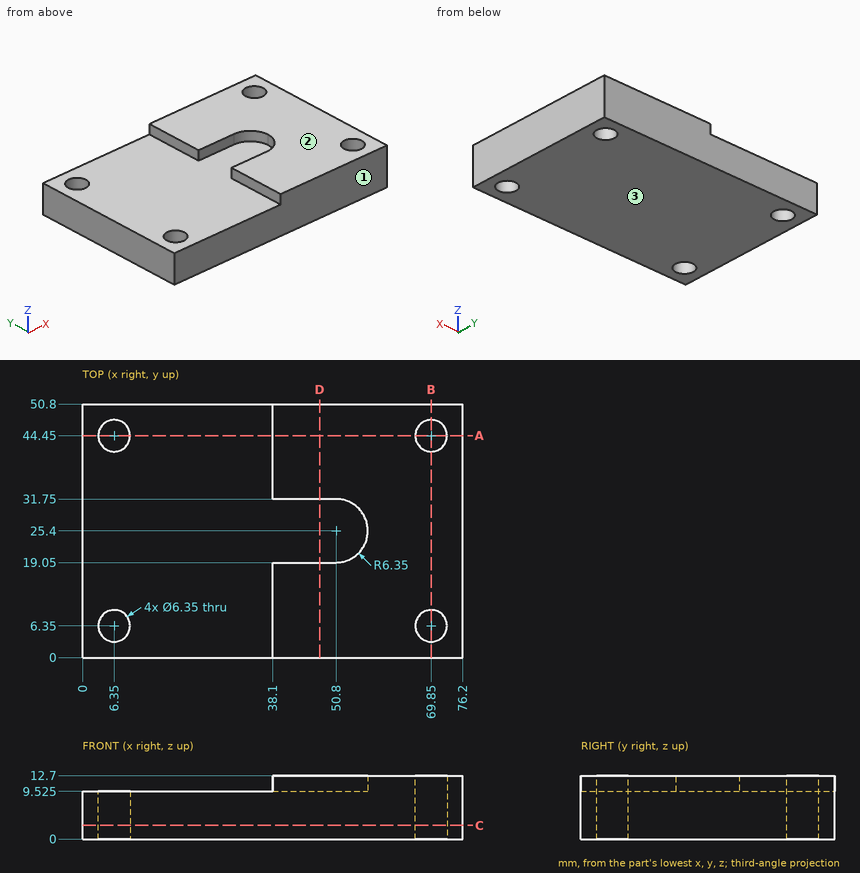
Part print with two shaded views. Sizes in mm from the minimum x, y, z corner. Give positions to 0.01 mm unless a question says otherwise; leave off trailing zeros. Order: outer loops, then holes, each group sorted by start corner. A loop starts at its lowest first (then second) coordinate and runs counter-clockwise, first axis right, second up.
(1) Mould opens along Z. For the marked faces 1, 2 and 3 say: released by +Z, released by -Z, zero draft, split by the parting line, or undercut.
(2) Flat gauge pin, fed straight in: pin 1 (2.5 mm diameter, centred on y = 45, z = 11.5, fed in from -X). Where does the tip first touch, or does it go through?
(3) Saw through at B-B, the plane x = 69.85. Give the cut face in (y, z) (3 decimals).
(4) Saw through at C-C, the plane z = 2.75. Give the cut face in (x, y) (3 decimals), then the cut area to 3 significant figures.
(5) Drill centre lines: L1, parallel to Y at x = 6.35, z = 7.5 (3 decimals); L2, parallel to X at y = 4, z = 2; L3, parallel to Y at x = 4.5, z = 4.75. Where is each one in solid material? Low to high.
(6) Saw through at A-A, the plane y = 44.45. Give the cut face in (x, z) (3 decimals).
(7) Saw through at D-D, the plane x = 47.5. Give the cut face in (y, z) (3 decimals).
Results found:
1. face 1: zero draft
1. face 2: released by +Z
1. face 3: released by -Z
2. pin 1: stops at x = 38.1
3. outline: (0, 0) - (3.175, 0) - (3.175, 12.7) - (0, 12.7) - close; (9.525, 0) - (41.275, 0) - (41.275, 12.7) - (9.525, 12.7) - close; (47.625, 0) - (50.8, 0) - (50.8, 12.7) - (47.625, 12.7) - close
4. outline: (0, 0) - (76.2, 0) - (76.2, 50.8) - (0, 50.8) - close; hole circle Ø6.35 at (6.35, 6.35); hole circle Ø6.35 at (6.35, 44.45); hole circle Ø6.35 at (69.85, 6.35); hole circle Ø6.35 at (69.85, 44.45)
4. area: 3,740 mm2
5. L1: y = 0 to 3.175, 9.525 to 41.275, 47.625 to 50.8
5. L2: x = 0 to 4.22, 8.48 to 67.72, 71.98 to 76.2
5. L3: y = 0 to 3.77, 8.93 to 41.87, 47.03 to 50.8
6. outline: (0, 0) - (3.175, 0) - (3.175, 9.525) - (0, 9.525) - close; (9.525, 0) - (66.675, 0) - (66.675, 12.7) - (38.1, 12.7) - (38.1, 9.525) - (9.525, 9.525) - close; (73.025, 0) - (76.2, 0) - (76.2, 12.7) - (73.025, 12.7) - close
7. outline: (0, 0) - (50.8, 0) - (50.8, 12.7) - (31.75, 12.7) - (31.75, 9.525) - (19.05, 9.525) - (19.05, 12.7) - (0, 12.7) - close
